from build123d import *

# Parameters (mm, degrees)
CROQUIS2_W              = 20
CROQUIS2_H              = 80
CROQUIS2_W_2            = 5.5
CROQUIS2_H_2            = 21
SALIENTE_EXTRUIR1_DEPTH = 5.5
CROQUIS3_W              = 5.5
CROQUIS3_H              = 21
SALIENTE_EXTRUIR2_DEPTH = 2.5
CROQUIS4_W              = 15.5
CROQUIS4_H              = 5.5
CROQUIS4_W_2            = 21
SALIENTE_EXTRUIR3_DEPTH = 2.5
CROQUIS5_W              = 5.5
CROQUIS5_H              = 21
SALIENTE_EXTRUIR4_DEPTH = 2.5
CROQUIS6_W              = 15.5
CROQUIS6_H              = 5.5
CROQUIS6_W_2            = 21
SALIENTE_EXTRUIR5_DEPTH = 2.5


with BuildPart() as part:
    # Croquis2 → Saliente-Extruir1 (new body)
    with BuildSketch(Plane.XY):
        Polygon((-47, 50), (-47, 31.5), (-50, 31.5), (-50, 10.5), (-47, 10.5), (-47, -10.5), (-50, -10.5), (-50, -31.5), (-47, -31.5), (-47, -50), (-31.5, -50), (-31.5, -47), (-10.5, -47), (-10.5, -50), (10.5, -50), (10.5, -47), (31.5, -47), (31.5, -50), (47, -50), (47, -31.5), (50, -31.5), (50, -10.5), (47, -10.5), (47, 10.5), (50, 10.5), (50, 31.5), (47, 31.5), (47, 50), (31.5, 50), (31.5, 47), (10.5, 47), (10.5, 50), (-10.5, 50), (-10.5, 47), (-31.5, 47), (-31.5, 50), align=None)
        with Locations((9.68, 0)):
            Rectangle(CROQUIS2_W, CROQUIS2_H, mode=Mode.SUBTRACT)
        with Locations((-24.16, 21)):
            Rectangle(CROQUIS2_W_2, CROQUIS2_H_2, mode=Mode.SUBTRACT)
        with Locations((-24.16, -21)):
            Rectangle(CROQUIS2_W_2, CROQUIS2_H_2, mode=Mode.SUBTRACT)
    extrude(amount=SALIENTE_EXTRUIR1_DEPTH)

    # Croquis3 → Saliente-Extruir2 (add)
    with BuildSketch(Plane.ZY.offset(50)):
        with Locations((2.75, -21)):
            Rectangle(CROQUIS3_W, CROQUIS3_H)
        with Locations((2.75, 21)):
            Rectangle(CROQUIS3_W, CROQUIS3_H)
    extrude(amount=SALIENTE_EXTRUIR2_DEPTH)

    # Croquis4 → Saliente-Extruir3 (add)
    with BuildSketch(Plane(origin=(0, 50, 0), x_dir=(1, 0, 0), z_dir=(0, 1, 0))):
        with Locations((39.25, -2.75)):
            Rectangle(CROQUIS4_W, CROQUIS4_H)
        with Locations((0, -2.75)):
            Rectangle(CROQUIS4_W_2, CROQUIS4_H)
        with Locations((-39.25, -2.75)):
            Rectangle(CROQUIS4_W, CROQUIS4_H)
    extrude(amount=SALIENTE_EXTRUIR3_DEPTH)

    # Croquis5 → Saliente-Extruir4 (add)
    with BuildSketch(Plane(origin=(50, 0, 0), x_dir=(0, 0, -1), z_dir=(1, 0, 0))):
        with Locations((-2.75, -21)):
            Rectangle(CROQUIS5_W, CROQUIS5_H)
        with Locations((-2.75, 21)):
            Rectangle(CROQUIS5_W, CROQUIS5_H)
    extrude(amount=SALIENTE_EXTRUIR4_DEPTH)

    # Croquis6 → Saliente-Extruir5 (add)
    with BuildSketch(Plane.XZ.offset(50)):
        with Locations((39.25, 2.75)):
            Rectangle(CROQUIS6_W, CROQUIS6_H)
        with Locations((0, 2.75)):
            Rectangle(CROQUIS6_W_2, CROQUIS6_H)
        with Locations((-39.25, 2.75)):
            Rectangle(CROQUIS6_W, CROQUIS6_H)
    extrude(amount=SALIENTE_EXTRUIR5_DEPTH)


solid = part.part
Check sheet for the modelled part. Datum: model origin and axes. Units: mm. A direction names the side the tool comes from. Coordinates: 2 decimals unless noted, no trailing zeros. Loops run counter-clockwise (first coordinate to the right, second up) from the corner with the lowest first, then second, coordinate; pieces in that order, holes last. Notation, with made-up numbers: (-19.5, 21) -> (5.5, 21) arc R23 ccw to (5.5, 56) -> close; hole circle Ø10 at (-14.75, 46). An arc over 180 degrees is marked (long way). Write item = value, one per line. Start each with the question number.
1. Tool access check on faces 1 (the flat face through (47, 0, 3)), 2 (the flat face through (-24, -10.5, 3)), 3 (the flat face through (10.5, -50, 3)), 4 (the flat face through (31.5, 50, 3)). Record the directions out of +Z, -Z, +X, -X, +Y, -Y that give a thin tool (end or side, any length) a straight path to the whole face; none if there is none.
2. Depth check by flat-ended pin: P1, Ø1.6, axis at x = 18, z = 4, coming from the -Y side; P2, Ø1.6, axis at y = 50, z = 2, coming from the -X side. Enter the tip coordinate at first touch or a pass-through.
3. Section check A-A on x = 4.5. Record the cut outline in (y, z), then the cut area to 4 significant figures.
4. Material ranges on line 1 (X direction, y = 26.5, z = 0.5); line 2 (Y direction, x = 18, z = 3.6); line 3 (Y direction, x = 1, z = 0.4), recorded low to high.
5. Section check C-C on z = 2.6. Give the number of separate pieces and of enclosed holes in the cut face, then the cut area to 3 significant figures.
6. Draft check along Y on faces 5 (the flat face through (-50, -31.5, 3)), 6 (the flat face through (50, -10.5, 3)), 7 (the flat face through (-47, 42, 3)). Enter one of: released by +Y, released by -Y, zero draft, split by the parting line, or undercut.
7. Section check B-B on y = -25.5. Record the cut outline in (x, z), then the cut area to 3 significant figures.
8. Section check D-D on x = -28.5. Record the cut outline in (y, z), then the cut area to 3 significant figures.
Responses:
q1.face_1 = +Z, -Z, +X
q1.face_2 = +Z, -Z
q1.face_3 = +Z, -Z, -Y
q1.face_4 = +Z, -Z, +Y
q2.P1 = -47
q2.P2 = -47
q3.outline = (-52.5, 0) -> (-40, 0) -> (-40, 5.5) -> (-52.5, 5.5) -> close; (40, 0) -> (52.5, 0) -> (52.5, 5.5) -> (40, 5.5) -> close
q3.area = 137.5 mm2
q4.line_1 = -52.5 to -26.91, -21.41 to -0.32, 19.68 to 52.5
q4.line_2 = -47 to -40, 40 to 47
q4.line_3 = -52.5 to -40, 40 to 52.5
q5.separate_pieces = 1
q5.enclosed_holes = 3
q5.area = 8,040 mm2
q6.face_5 = released by -Y
q6.face_6 = undercut
q6.face_7 = zero draft
q7.outline = (-52.5, 0) -> (-26.91, 0) -> (-26.91, 5.5) -> (-52.5, 5.5) -> close; (-21.41, 0) -> (-0.32, 0) -> (-0.32, 5.5) -> (-21.41, 5.5) -> close; (19.68, 0) -> (52.5, 0) -> (52.5, 5.5) -> (19.68, 5.5) -> close
q7.area = 437 mm2
q8.outline = (-47, 0) -> (47, 0) -> (47, 5.5) -> (-47, 5.5) -> close
q8.area = 517 mm2
